Input: part model. Units: mm. Frame: model coordinates. A direction names the side the tool comes from. Give positions to 0.01 mm unless a question says otherwise; leave off trailing zeros. Write each loop counter-clockwise with the first axis right and the second up, starting at its lowest first coordinate (ties: lowest second). Pieces come first, ordered by that corner, then holes.
```python
from build123d import *

# Parameters (mm, degrees)
SKETCH_R        = 11.5
PAD_DEPTH       = 3
SKETCH001_R     = 10
PAD001_DEPTH    = 10
SKETCH002_R     = 11.5
PAD002_DEPTH    = 3
SKETCH003_R     = 2.6
POCKET_DEPTH    = 16
SKETCH004_R     = 6.975
POCKET001_DEPTH = 5
SKETCH005_R     = 6.975
POCKET002_DEPTH = 5


with BuildPart() as part:
    # Sketch → Pad (new body)
    with BuildSketch(Plane.XY):
        Circle(SKETCH_R)
    extrude(amount=PAD_DEPTH)

    # Sketch001 (on Face3 of Pad) → Pad001 (join)
    with BuildSketch(Plane.XY.offset(3)):
        Circle(SKETCH001_R)
    extrude(amount=PAD001_DEPTH)

    # Sketch002 (on Face5 of Pad001) → Pad002 (join)
    with BuildSketch(Plane.XY.offset(13)):
        Circle(SKETCH002_R)
    extrude(amount=PAD002_DEPTH)

    # Sketch003 (on Face3 of Pad002) → Pocket (cut)
    with BuildSketch(Plane.XY.offset(16)):
        Circle(SKETCH003_R)
    extrude(amount=-POCKET_DEPTH, mode=Mode.SUBTRACT)

    # Sketch004 (on Face3 of Pocket) → Pocket001 (cut)
    with BuildSketch(Plane.XY.offset(16)):
        Circle(SKETCH004_R)
    extrude(amount=-POCKET001_DEPTH, mode=Mode.SUBTRACT)

    # Sketch005 (on Face10 of Pocket001) → Pocket002 (cut)
    with BuildSketch(Plane(origin=(0, 0, 0), x_dir=(1, 0, 0), z_dir=(0, 0, -1))):
        Circle(SKETCH005_R)
    extrude(amount=-POCKET002_DEPTH, mode=Mode.SUBTRACT)


solid = part.part
```
Q1. Access query for faces 5 (the cylindrical face through (-1.5, 11.4, 1.5)), 6 (the flat face through (0, -8, 0)), 7 (the flat face through (-9, 5, 13)), 8 (the cylindrical face through (-1.51, 6.81, 2.46)), 9 (the cylindrical face through (-1.51, -6.81, 13.54)). Directions: +Z, -Z, +X, -X, +Y, -Y. A direction counts if a zero-diameter tool reaches every point of the face in a straight line with its end or side. Return the directions, or none.
Q2. Pin query (flat end, axial travel): pin 1 (11 mm diameter, centred on x = 2.5, y = 3, fed in from -Z); pin 2 (6 mm diameter, centred on y = 9, z = 6.5, fed in from -X); pin 3 (8.5 mm diameter, centred on x = 0, y = 0, fed in from +Z); pin 4 (1.5 mm diameter, centred on x = 4.5, z = 8, fed in from +Y). Return the tip coordinate at first contact, or that it passes through.
Q3. Section C-C, the plane z = 8. Return the cut outline in (x, y), then the cut area to 3 significant figures.
Q4. Material intervals for line 1 along Y through (x, z) = (0, 2.5) (3 decimals); line 2 along Y through (x, z) = (0, 7.45); line 3 along Z through (x, y) = (10.75, 4), sorted ascending.
Q5. Section A-A, the plane x = 0. Return the cut outline in (y, z) (3 decimals), then the cut area to 3 significant figures.
Q6. Mould query, pull axis Z, two halves, no side actions, for faces 1 (the flat face through (3, 0, 5)), 2 (the cylindrical face through (-1.5, 11.4, 14.5)), 3 (the flat face through (-9, 5, 3)), 4 (the flat face through (0, -8, 16)). Classes: +Z half, -Z half, draft (parallel to the pull), parting line (faces both ways), or undercut.
Q7. Section D-D, the plane x = -5.25. Return the cut outline in (y, z).
Solutions:
1. face 5: +Z, -Z
1. face 6: -Z, +X, -X, +Y, -Y
1. face 7: none
1. face 8: -Z
1. face 9: +Z
2. pin 1: stops at z = 0
2. pin 2: stops at x = -8
2. pin 3: stops at z = 11
2. pin 4: stops at y = 9.27
3. outline: circle Ø20 at (0, 0); hole circle Ø5.2 at (0, 0)
3. area: 293 mm2
4. line 1: y = -11.5 to -6.975, 6.975 to 11.5
4. line 2: y = -10 to -2.6, 2.6 to 10
4. line 3: z = 0 to 3, 13 to 16
5. outline: (-11.5, 0) - (-6.975, 0) - (-6.975, 5) - (-2.6, 5) - (-2.6, 11) - (-6.975, 11) - (-6.975, 16) - (-11.5, 16) - (-11.5, 13) - (-10, 13) - (-10, 3) - (-11.5, 3) - close; (2.6, 5) - (6.975, 5) - (6.975, 0) - (11.5, 0) - (11.5, 3) - (10, 3) - (10, 13) - (11.5, 13) - (11.5, 16) - (6.975, 16) - (6.975, 11) - (2.6, 11) - close
5. area: 167 mm2
6. face 1: -Z half
6. face 2: draft
6. face 3: undercut
6. face 4: +Z half
7. outline: (-10.23, 0) - (-4.59, 0) - (-4.59, 5) - (4.59, 5) - (4.59, 0) - (10.23, 0) - (10.23, 3) - (8.51, 3) - (8.51, 13) - (10.23, 13) - (10.23, 16) - (4.59, 16) - (4.59, 11) - (-4.59, 11) - (-4.59, 16) - (-10.23, 16) - (-10.23, 13) - (-8.51, 13) - (-8.51, 3) - (-10.23, 3) - close
